from build123d import *

# Parameters (mm, degrees)
BOSS_EXTRUDE1_DEPTH           = 5
CHAMFER1_SIZE                 = 2
SKETCH4_W                     = 12
SKETCH4_H                     = 3
BOSS_EXTRUDE2_DEPTH           = 11.35
BOSS_EXTRUDE3_DEPTH           = 4
BOSS_EXTRUDE4_DEPTH           = 11.35
CHAMFER2_START                = 116.672618896
CHAMFER2_OUTLINE_W            = 5
CHAMFER2_OUTLINE_H            = 5.65
CHAMFER2_DEPTH                = 2.327381104
CUT_EXTRUDE2_DEPTH            = 2
BOSS_EXTRUDE5_DEPTH           = 9
BOSS_EXTRUDE6_DEPTH           = 12
SKETCH11_W                    = 3
SKETCH11_H                    = 100.242640687
BOSS_EXTRUDE7_DEPTH           = 9
CHAMFER3_SIZE                 = 2
SKETCH12_W                    = 21
SKETCH12_H                    = 5
CUT_EXTRUDE3_DEPTH            = 9
CHAMFER5_SIZE                 = 4.996701125
CHAMFER5_SIZE_2               = 2.33
SKETCH13_W                    = 12
SKETCH13_H                    = 11.35
CUT_EXTRUDE4_DEPTH            = 117
SKETCH14_W                    = 3
SKETCH14_H                    = 11.35
BOSS_EXTRUDE8_DEPTH           = 7
BOSS_EXTRUDE9_START           = 85.242641
SKETCH14_2_W                  = 3
SKETCH14_2_H                  = 11.35
BOSS_EXTRUDE9_DEPTH           = 8
SKETCH15_W                    = 9
SKETCH15_H                    = 92
CUT_EXTRUDE5_DEPTH            = 10
BOSS_EXTRUDE10_START          = -9
SKETCH16_W                    = 62
SKETCH16_H                    = 3
BOSS_EXTRUDE10_DEPTH          = 31.5
BOSS_EXTRUDE12_DEPTH          = 6
SKETCH18_W                    = 50
SKETCH18_H                    = 86
CUT_EXTRUDE6_DEPTH            = 6
CUT_EXTRUDE7_DEPTH            = 3
SKETCH20_W                    = 6
SKETCH20_H                    = 98
CUT_EXTRUDE8_DEPTH            = 3
BOSS_EXTRUDE13_DEPTH          = 10.5
SKETCH22_W                    = 3
SKETCH22_H                    = 92
BOSS_EXTRUDE14_DEPTH          = 3
CUT_EXTRUDE9_START            = -2
CUT_EXTRUDE9_DEPTH            = 10
CUT_EXTRUDE10_DEPTH           = 9
SKETCH25_W                    = 9.5
SKETCH25_H                    = 30
BOSS_EXTRUDE15_DEPTH          = 10
CSK_FOR_M4_SFHCS2_D           = 4
CSK_FOR_M4_SFHCS2_DEPTH       = 13
CSK_FOR_M4_SFHCS2_CSINK_D     = 7.9
CSK_FOR_M4_SFHCS2_CSINK_ANGLE = 90
CSK_FOR_M4_SFHCS2_TIP         = 1.201721238
CHAMFER6_SIZE                 = 2
CHAMFER6_SIZE_2               = 4.289013841
SKETCH30_W                    = 56
SKETCH30_H                    = 25.5
CUT_EXTRUDE11_DEPTH           = 18.5
SKETCH32_W                    = 30
SKETCH32_H                    = 6
CUT_EXTRUDE13_DEPTH           = 10
CSK_FOR_M4_SFHCS3_D           = 4
CSK_FOR_M4_SFHCS3_DEPTH       = 19
CSK_FOR_M4_SFHCS3_CSINK_D     = 7.9
CSK_FOR_M4_SFHCS3_CSINK_ANGLE = 90
CSK_FOR_M4_SFHCS3_TIP         = 1.201721238
F_4_0MM_DOWEL_HOLE1_D         = 4


with BuildPart() as part:
    # Sketch2 → Boss-Extrude1 (new body)
    with BuildSketch(Plane.XY):
        Polygon((-45, 122), (-45, 0.197559457), (-24, -13.44), (24, -13.44), (45, 0.197559457), (45, 122), align=None)
    extrude(amount=BOSS_EXTRUDE1_DEPTH)

    # Chamfer1
    chamfer1_edges = [part.edges().sort_by_distance(p)[0] for p in [
        (45, 122, 2.5),
        (-45, 122, 2.5),
    ]]
    chamfer(chamfer1_edges, length=CHAMFER1_SIZE)

    # Sketch4 → Boss-Extrude2 (add)
    with BuildSketch(Plane.XY.offset(5)):
        Polygon((-45, 120), (-43, 122), (-33, 122), (-33, 119), (-41.757359313, 119), (-42, 118.757359313), (-45, 118.757359313), align=None)
        with Locations((-39, 17.257359313)):
            Rectangle(SKETCH4_W, SKETCH4_H)
        Polygon((0, 122), (30, 122), (30, 108), (27, 108), (27, 119), (0, 119), align=None)
        Polygon((0, 15.757359313), (30, 15.757359313), (30, 29.757359313), (27, 29.757359313), (27, 18.757359313), (0, 18.757359313), align=None)
    extrude(amount=BOSS_EXTRUDE2_DEPTH)

    # Sketch5 → Boss-Extrude3 (add)
    with BuildSketch(Plane.XY.offset(16.35)):
        Polygon((45, 15.757359313), (-45, 15.757359313), (-45, 120), (-43, 122), (45, 122), align=None)
    extrude(amount=BOSS_EXTRUDE3_DEPTH)

    # Sketch6 → Boss-Extrude4 (add)
    with BuildSketch(Plane.XY.offset(5)):
        Polygon((38, 122), (43, 122), (45, 120), (45, 115), (42, 115), (42, 118.757359313), (41.757359313, 119), (38, 119), align=None)
        Polygon((45, 15.757359313), (39, 15.757359313), (39, 18.757359313), (42, 18.757359313), (42, 21.757359313), (45, 21.757359313), align=None)
    extrude(amount=BOSS_EXTRUDE4_DEPTH)

    # Chamfer2: read off the stored shape, not the designer's step
    # Chamfer2 outline → Chamfer2 (cut)
    with BuildSketch(Plane(origin=(0, 0, 0), x_dir=(0.7071067811865474, -0.7071067811865477, 0), z_dir=(0.7071067811865476, 0.7071067811865476, 0)).offset(CHAMFER2_START)):
        with Locations((-54.5, -19.175)):
            Rectangle(CHAMFER2_OUTLINE_W, CHAMFER2_OUTLINE_H)
    extrude(amount=CHAMFER2_DEPTH, mode=Mode.SUBTRACT)

    # Sketch8 → Cut-Extrude2 (cut)
    with BuildSketch(Plane.XY.offset(20.35)):
        Polygon((-45, 15.757359313), (-37, 15.757359313), (-37, 122), (-43, 122), (-45, 120), align=None)
    extrude(amount=-CUT_EXTRUDE2_DEPTH, mode=Mode.SUBTRACT)

    # Sketch9 → Boss-Extrude5 (add)
    with BuildSketch(Plane.XY.offset(20.35)):
        Polygon((-37, 18.757359313), (42, 18.757359313), (42, 118.757359313), (41.757359313, 119), (-37, 119), (-37, 122), (43, 122), (45, 120), (45, 15.757359313), (-37, 15.757359313), align=None)
    extrude(amount=BOSS_EXTRUDE5_DEPTH)

    # Sketch10 → Boss-Extrude6 (add)
    with BuildSketch(Plane.ZY.offset(37)):
        Polygon((18.35, 15.757359313), (29.35, 15.757359313), (29.35, 18.757359313), (20.35, 18.757359313), (20.35, 119), (29.35, 119), (29.35, 122), (18.35, 122), align=None)
    extrude(amount=BOSS_EXTRUDE6_DEPTH)

    # Sketch11 → Boss-Extrude7 (add)
    with BuildSketch(Plane.XY.offset(20.35)):
        with Locations((-47.5, 68.878679657)):
            Rectangle(SKETCH11_W, SKETCH11_H)
    extrude(amount=BOSS_EXTRUDE7_DEPTH)

    # Chamfer3
    chamfer3_edges = [part.edges().sort_by_distance(p)[0] for p in [
        (-49, 15.757359313, 23.85),
        (-49, 122, 23.85),
    ]]
    chamfer(chamfer3_edges, length=CHAMFER3_SIZE)

    # Sketch12 → Cut-Extrude3 (cut)
    with BuildSketch(Plane(origin=(0, 18.757359313, 0), x_dir=(1, 0, 0), z_dir=(0, 1, 0))):
        with Locations((27.5, -22.85)):
            Rectangle(SKETCH12_W, SKETCH12_H)
    extrude(amount=-CUT_EXTRUDE3_DEPTH, mode=Mode.SUBTRACT)

    # Chamfer5
    # the kernel refuses this chamfer: 4.996701125, 2.33 mm, written as the material it takes off along each edge
    with BuildSketch(Plane(origin=(38, 18.757359313, 20.35), x_dir=(1, 0, 0), z_dir=(0, 0, 1))) as chamfer5_piece_1_section:
        Polygon((CHAMFER5_SIZE, 0), (0, -CHAMFER5_SIZE_2), (0, 0), align=None)
    chamfer5_piece_1 = extrude(amount=5, mode=Mode.PRIVATE)
    chamfer5_piece_1 = split(chamfer5_piece_1, bisect_by=Plane(origin=(42, 18.757359313, 20.35), z_dir=(-1, 0, 0)), keep=Keep.TOP, mode=Mode.PRIVATE)
    add(chamfer5_piece_1, mode=Mode.SUBTRACT)
    with BuildSketch(Plane(origin=(17, 18.757359313, 25.35), x_dir=(-1, 0, 0), z_dir=(0, 0, -1))) as chamfer5_piece_2:
        Polygon((CHAMFER5_SIZE, 0), (0, -CHAMFER5_SIZE_2), (0, 0), align=None)
    extrude(amount=5, mode=Mode.SUBTRACT)

    # Sketch13 → Cut-Extrude4 (cut)
    with BuildSketch(Plane(origin=(0, 122, 0), x_dir=(1, 0, 0), z_dir=(0, 1, 0))):
        with Locations((36, -10.675)):
            Rectangle(SKETCH13_W, SKETCH13_H)
    extrude(amount=-CUT_EXTRUDE4_DEPTH, mode=Mode.SUBTRACT)

    # Sketch14 → Boss-Extrude8 (add)
    with BuildSketch(Plane.XZ.offset(-115)):
        with Locations((43.5, 10.675)):
            Rectangle(SKETCH14_W, SKETCH14_H)
    extrude(amount=BOSS_EXTRUDE8_DEPTH)

    # Sketch14<2> → Boss-Extrude9 (add)
    with BuildSketch(Plane.XZ.offset(-115).offset(BOSS_EXTRUDE9_START)):
        with Locations((43.5, 10.675)):
            Rectangle(SKETCH14_2_W, SKETCH14_2_H)
    extrude(amount=BOSS_EXTRUDE9_DEPTH)

    # Sketch15 → Cut-Extrude5 (cut)
    with BuildSketch(Plane.ZY.offset(49)):
        with Locations((24.85, 73)):
            Rectangle(SKETCH15_W, SKETCH15_H)
    extrude(amount=-CUT_EXTRUDE5_DEPTH, mode=Mode.SUBTRACT)

    # Sketch16 → Boss-Extrude10 (add)
    with BuildSketch(Plane.XY.offset(29.35).offset(BOSS_EXTRUDE10_START)):
        Polygon((13, 122), (13, 119), (-49, 119), (-49, 120), (-47, 122), align=None)
        with Locations((-18, 25.5)):
            Rectangle(SKETCH16_W, SKETCH16_H)
    extrude(amount=BOSS_EXTRUDE10_DEPTH)

    # Sketch17 → Boss-Extrude12 (add)
    with BuildSketch(Plane.XY.offset(51.85)):
        Polygon((-49, 119), (-49, 27), (-49, 24), (13, 24), (13, 27), (13, 119), (13, 122), (-47, 122), (-49, 120), align=None)
    extrude(amount=BOSS_EXTRUDE12_DEPTH)

    # Sketch18 → Cut-Extrude6 (cut)
    with BuildSketch(Plane.XY.offset(57.85)):
        with Locations((-18, 73)):
            Rectangle(SKETCH18_W, SKETCH18_H)
    extrude(amount=-CUT_EXTRUDE6_DEPTH, mode=Mode.SUBTRACT)

    # Sketch19 → Cut-Extrude7 (cut)
    with BuildSketch(Plane.XY.offset(57.85)):
        Polygon((10, 119), (-45.757359313, 119), (-46, 118.757359313), (-46, 27), (10, 27), align=None)
    extrude(amount=-CUT_EXTRUDE7_DEPTH, mode=Mode.SUBTRACT)

    # Sketch20 → Cut-Extrude8 (cut)
    with BuildSketch(Plane(origin=(13, 0, 0), x_dir=(0, 0, -1), z_dir=(1, 0, 0))):
        with Locations((-54.85, 73)):
            Rectangle(SKETCH20_W, SKETCH20_H)
    extrude(amount=-CUT_EXTRUDE8_DEPTH, mode=Mode.SUBTRACT)

    # Sketch21 → Boss-Extrude13 (add)
    with BuildSketch(Plane(origin=(10, 0, 0), x_dir=(0, 0, -1), z_dir=(1, 0, 0))):
        Polygon((-57.85, 27), (-57.85, 24), (-51.85, 24), (-51.85, 27), (-51.85, 119), (-51.85, 122), (-57.85, 122), (-57.85, 119), (-54.85, 119), (-54.85, 27), align=None)
    extrude(amount=BOSS_EXTRUDE13_DEPTH)

    # Sketch22 → Boss-Extrude14 (add)
    with BuildSketch(Plane.XY.offset(54.85)):
        with Locations((19, 73)):
            Rectangle(SKETCH22_W, SKETCH22_H)
    extrude(amount=BOSS_EXTRUDE14_DEPTH)

    # Sketch23 → Cut-Extrude9 (cut)
    with BuildSketch(Plane.XY.offset(20.35).offset(CUT_EXTRUDE9_START)):
        Polygon((13, 15.757359313), (13, 119), (41.757359313, 119), (42, 118.757359313), (42, 15.757359313), align=None)
    extrude(amount=CUT_EXTRUDE9_DEPTH, mode=Mode.SUBTRACT)

    # Sketch24 → Cut-Extrude10 (cut)
    with BuildSketch(Plane.XY.offset(29.35)):
        Polygon((43, 15.757359313), (42, 18.757359313), (-46, 18.757359313), (-46, 24), (-49, 24), (-49, 17.757359313), (-47, 15.757359313), align=None)
    extrude(amount=-CUT_EXTRUDE10_DEPTH, mode=Mode.SUBTRACT)

    # Sketch25 → Boss-Extrude15 (add)
    with BuildSketch(Plane(origin=(0, 0, 0), x_dir=(-1, 0, 0), z_dir=(0, 0, -1))):
        with Locations((30.75, 107)):
            Rectangle(SKETCH25_W, SKETCH25_H)
        with Locations((-30.75, 107)):
            Rectangle(SKETCH25_W, SKETCH25_H)
    extrude(amount=BOSS_EXTRUDE15_DEPTH)

    # CSK for M4 SFHCS2
    with Locations(Plane(origin=(-695.683007616, 1385.247292614, 5), x_dir=(1, 0, 0), z_dir=(0, 0, 1))):
        with Locations((678.683007616, -1390.467292614), (712.683007616, -1390.467292614)):
            CounterSinkHole(CSK_FOR_M4_SFHCS2_D / 2, CSK_FOR_M4_SFHCS2_CSINK_D / 2, depth=CSK_FOR_M4_SFHCS2_DEPTH, counter_sink_angle=CSK_FOR_M4_SFHCS2_CSINK_ANGLE)
            with Locations((0, 0, -(CSK_FOR_M4_SFHCS2_DEPTH + CSK_FOR_M4_SFHCS2_TIP / 2))):  # 118° drill point
                Cone(0, CSK_FOR_M4_SFHCS2_D / 2, CSK_FOR_M4_SFHCS2_TIP, mode=Mode.SUBTRACT)

    # Chamfer6
    # the kernel refuses this chamfer: 4.289013841, 2 mm, written as the material it adds along each edge
    with BuildSketch(Plane(origin=(-45, 131.112729659, 18.35), x_dir=(0, 0, -1), z_dir=(0, -1, 0))) as chamfer6_piece_1_section:
        Polygon((CHAMFER6_SIZE, 0), (0, -CHAMFER6_SIZE_2), (0, 0), align=None)
    chamfer6_piece_1 = extrude(amount=115.355370346, mode=Mode.PRIVATE)
    chamfer6_piece_1 = split(chamfer6_piece_1, bisect_by=Plane(origin=(-49, 131.112729659, 18.35), z_dir=(1, 0, 0)), keep=Keep.TOP, mode=Mode.PRIVATE)
    chamfer6_piece_1 = split(chamfer6_piece_1, bisect_by=Plane(origin=(-39.443635171, 125.556364829, 18.35), z_dir=(0.7071067811865476, -0.7071067811865476, 0)), keep=Keep.TOP, mode=Mode.PRIVATE)
    chamfer6_piece_1 = split(chamfer6_piece_1, bisect_by=Plane(origin=(-103.677685173, 72.435044486, 18.35), z_dir=(0.7071067811865476, 0.7071067811865476, 0)), keep=Keep.TOP, mode=Mode.PRIVATE)
    add(chamfer6_piece_1)

    # Sketch30 → Cut-Extrude11 (cut)
    with BuildSketch(Plane(origin=(-695.683007616, 24, -941.083024415), x_dir=(1, 0, 0), z_dir=(0, -1, 0))):
        with Locations((677.683007616, 980.183024415)):
            Rectangle(SKETCH30_W, SKETCH30_H)
    extrude(amount=-CUT_EXTRUDE11_DEPTH, mode=Mode.SUBTRACT)

    # Sketch32 → Cut-Extrude13 (cut)
    with BuildSketch(Plane(origin=(0, 122, 0), x_dir=(1, 0, 0), z_dir=(0, 1, 0))):
        with Locations((-34, -32.35)):
            Rectangle(SKETCH32_W, SKETCH32_H)
    extrude(amount=-CUT_EXTRUDE13_DEPTH, mode=Mode.SUBTRACT)

    # CSK for M4 SFHCS3
    with Locations(Plane(origin=(45, 1385.247292614, -941.083024415), x_dir=(0, 1, 0), z_dir=(1, 0, 0))):
        with Locations((-1278.247292614, 936.083024415)):
            CounterSinkHole(CSK_FOR_M4_SFHCS3_D / 2, CSK_FOR_M4_SFHCS3_CSINK_D / 2, depth=CSK_FOR_M4_SFHCS3_DEPTH, counter_sink_angle=CSK_FOR_M4_SFHCS3_CSINK_ANGLE)
            with Locations((0, 0, -(CSK_FOR_M4_SFHCS3_DEPTH + CSK_FOR_M4_SFHCS3_TIP / 2))):  # 118° drill point
                Cone(0, CSK_FOR_M4_SFHCS3_D / 2, CSK_FOR_M4_SFHCS3_TIP, mode=Mode.SUBTRACT)

    # Ø4.0mm Dowel Hole1 (through all)
    with Locations(Plane.ZY.offset(35.5)):
        with Locations((-5, 107)):
            Hole(F_4_0MM_DOWEL_HOLE1_D / 2)


solid = part.part
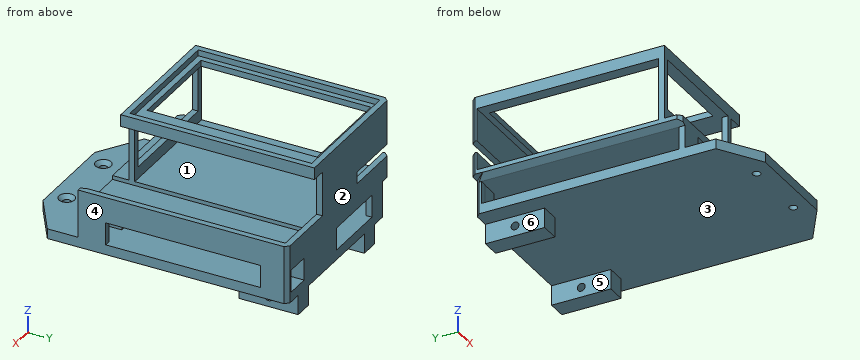
The model under review builds one solid part; all positions refer to its coordinate system, in mm. Face numbers are marked on the shaded views. A direction names the side the tool comes from. Round coordinates to 2 decimals unless told otherwise and drop trailing zeros. Order: outer loops, then holes, each group sorted by start corner. A loop starts at its lowest first (then second) coordinate and runs counter-clockwise, first axis right, second up. Notation, with made-up numbers: (10.25, -8) -> (36.25, -8) arc R29 ccw to (36.25, 22) -> close; hole circle Ø10 at (51, 67.5). An arc over 180 degrees is marked (long way). Use CSV: the item, a comma, the result in double quotes. Start each with the question number.
(1) Mouldability with a two-part tool opening along Y and no side actions: class the marked faces 1, 2 and 3 as pulls with the +Y half, pulls with the -Y half, needs draft (parallel to the pull), parting line crosses it, or undercut.
(2) Consider section B-B on x = -17. State how many separate pieces and enclosed holes the cut face has, and give its area (3 significant figures).
(3) Consider section C-C on y = 70.5. Write out the cut boundary in (x, z), and give its area (3 significant figures).
(4) Insertion check: pin 1 (3.5 mm diameter, centred on x = -44, z = 10, fed in from -Y); pin 2 (1.5 mm diameter, centred on y = 94, z = -0.5, fed in from -X); pin 3 (1.5 mm diameter, centred on y = 120.5, z = 45, fed in from +X); pin 4 (3.5 mm diameter, centred on y = 107, z = -5, fed in from -X) (3 decimals). Each pin has a flat end and moves straight along its axis. Give the tip position at first contact, or say it passes through.
(5) Wall thickness on probe 1 along Z at (x, y) = (10, 62.5); probe 2 along Z at (x, y) = (15.5, 95); probe 3 along Z at (x, y) = (-16, 102): over which ranges is each line inside the solid? List them lowest first. Write a range as from..to.
(6) Tool access review of the marked faces 4, 5 and 6: name each direction out of +Z, -Z, +X, -X, +Y, -Y from which nothing blocks a thin tool from reaching the whole face with its end or side.
(7) Consider section A-A on z = -5. Write out the cut boundary in (x, y).
Responses:
1,face 1,"undercut"
1,face 2,"pulls with the +Y half"
1,face 3,"needs draft"
2,separate pieces,"4"
2,enclosed holes,"0"
2,area,"1,240 mm²"
3,outline,"(-49, 18.22) -> (-45, 16.35) -> (45, 16.35) -> (45, 29.35) -> (42, 29.35) -> (42, 18.35) -> (13, 18.35) -> (13, 20.35) -> (-49, 20.35) -> close; (-49, 51.85) -> (-43, 51.85) -> (-43, 54.85) -> (-46, 54.85) -> (-46, 57.85) -> (-49, 57.85) -> close; (-45, 0) -> (45, 0) -> (45, 5) -> (-45, 5) -> close; (7, 51.85) -> (20.5, 51.85) -> (20.5, 57.85) -> (17.5, 57.85) -> (17.5, 54.85) -> (7, 54.85) -> close"
3,area,"868 mm²"
4,pin 1,"y = 15.76"
4,pin 2,"x = -45"
4,pin 3,"x = 13"
4,pin 4,"through"
5,probe 1,"0..5, 16.35..20.35, 51.85..54.85"
5,probe 2,"0..5, 16.35..18.35, 51.85..54.85"
5,probe 3,"0..5, 16.35..20.35"
6,face 4,"+Z, -Z, +X, +Y, -Y"
6,face 5,"-Z, +Y, -Y"
6,face 6,"-Z, -X, +Y, -Y"
7,outline,"(-35.5, 92) -> (-26, 92) -> (-26, 105) -> (-35.5, 105) -> close; (-35.5, 109) -> (-26, 109) -> (-26, 122) -> (-35.5, 122) -> close; (26, 92) -> (35.5, 92) -> (35.5, 105) -> (26, 105) -> close; (26, 109) -> (35.5, 109) -> (35.5, 122) -> (26, 122) -> close"
